The drawing under review shows one solid part. Ordinate dimensions are in mm from its lowest x, y, z. Give positions to 0.01 mm unless a question says otherwise; leave off trailing zeros. Loops run counter-clockwise (first coordinate to the right, second up) from the corner with the lowest first, then second, coordinate; pieces in that order, holes last. Notation, with made-up numbers: M 59.25,-30.75 L 87.25,-30.75 A23 cw 87.25,-16.75 Z; hole C 81.25,35.25 d3. An arc over 180 degrees is marked long. Write item = value, one per line. Start each with the question number.
1. Wall thickness on line 1 along X through (y, z) = (11.5, 1.2); line 2 along X through (y, z) = (10.5, 1.7); line 3 along Y through (x, z) = (39.5, 1.1): over which ranges is each line inside the solid? List them lowest first. Write a range as from..to.
2. We need section A-A on x = 20. Give the boundary of the cut face in (y, z).
3. For pin 1 (3.5 mm diameter, centred on x = 60, y = 30, fed in from +Z), flat-tipped, find the tip position at first contact; note if it passes through.
4. We need section B-B on y = 30. Give the boundary of the cut face in (x, z), then the cut area to 3 significant figures.
5. We need section C-C on z = 1.2. Give the boundary of the cut face in (x, y), then the cut area to 3 significant figures.
6. We need section D-D on x = 60. Give the boundary of the cut face in (y, z).
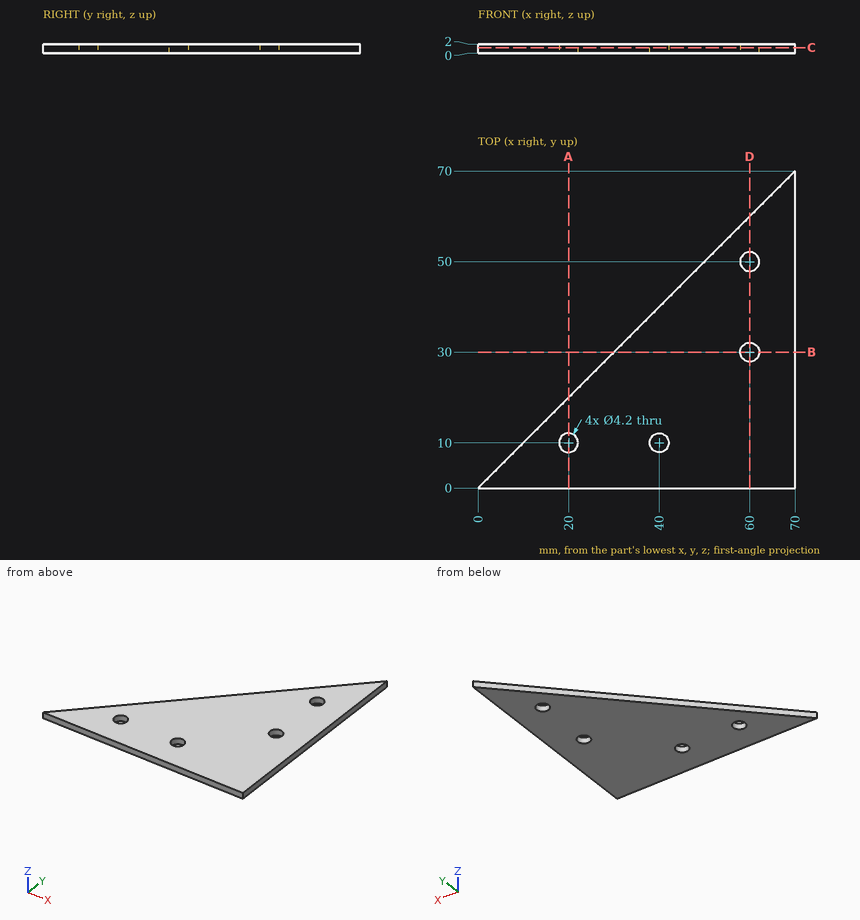
Final values:
q1.line_1 = 11.5..18.53, 21.47..38.53, 41.47..70
q1.line_2 = 10.5..17.96, 22.04..37.96, 42.04..70
q1.line_3 = 0..7.96, 12.04..39.5
q2.outline = M 0,0 L 7.9,0 L 7.9,2 L 0,2 Z; M 12.1,0 L 20,0 L 20,2 L 12.1,2 Z
q3.pin_1 = through
q4.outline = M 30,0 L 57.9,0 L 57.9,2 L 30,2 Z; M 62.1,0 L 70,0 L 70,2 L 62.1,2 Z
q4.area = 71.6 mm²
q5.outline = M 0,0 L 70,0 L 70,70 Z; hole C 20,10 d4.2; hole C 40,10 d4.2; hole C 60,30 d4.2; hole C 60,50 d4.2
q5.area = 2,390 mm²
q6.outline = M 0,0 L 27.9,0 L 27.9,2 L 0,2 Z; M 32.1,0 L 47.9,0 L 47.9,2 L 32.1,2 Z; M 52.1,0 L 60,0 L 60,2 L 52.1,2 Z
